Input: part model. Units: mm. Frame: model coordinates. A direction names the side the tool comes from. Round coordinates to 2 decimals unless told otherwise and drop trailing zeros. Loops run counter-clockwise (first coordinate to the right, second up) from the corner with the lowest first, then second, coordinate; pieces in that order, holes last.
(1) Cut plane C-C, the plane y = 0. Output: boundary loops of the cut face in (x, z).
(2) Line query: line 1 (Y direction, x = 0.6, z = 0); line 2 (Z direction, x = -1.5, y = 0.5); line 3 (Y direction, x = -1.5, z = -290). Output: solid intervals per line, ascending.
(3) First-contact query: pin 1 Ø2 at (x, z) = (0, -53) entering from +Y; pin 2 Ø6 at (x, z) = (0.5, -205.5) entering from +Y; pin 3 Ø3 at (x, y) = (-0.5, -20.5) entering from +Z. Flat tips, straight axial feed; report the tip coordinate or a pass-through.
(4) Access query for faces 3 (the face through (0.077, -99.847, -256.535)), 4 (the face through (3.007, -2.733, 116.812)), 5 (the face through (-2.97, 1.37, -566.71)), 6 (the face through (-0.04, -91.19, -255.66)). Directions: +Z, -Z, +X, -X, +Y, -Y. A direction counts if a zero-diameter tool reaches every point of the face in a straight line with its end or side. Return the directions, or none.
(5) Cut plane B-B, the plane z = 0. Output: boundary loops of the cut face in (x, y).
(6) Cut plane A-A, the plane x = 1. Output: boundary loops of the cut face in (y, z), and give its area (3 significant figures).
(7) Draft query along Z for faces 1 (the face through (0.08, 99.15, -263.47)), 2 (the face through (-2.97, -2.73, 116.69)). Return one class per face: released by +Z, released by -Z, zero draft, split by the parting line, or undercut.
from build123d import *


with BuildPart() as part:
    # 扫描1: sweep along a path in 草图1
    with BuildLine(Plane(origin=(0, 0, 0), x_dir=(0, 0, -1), z_dir=(1, 0, 0))) as sweep_1_path:
        Line((12.5, 124.373429638), (507.5, 74.624057783))
        ThreePointArc((507.5, 74.624057783), (575, 0), (507.5, -74.624057783))
        Line((507.5, -74.624057783), (12.5, -124.373429638))
        ThreePointArc((12.5, -124.373429638), (-125, 0), (12.5, 124.373429638))
    # 草图2 → 扫描1 (sweep)
    with BuildSketch(Plane.XY):
        Polygon((-5.5, 125), (5.5, 125), (2.840143071, 116.3), (-2.840143071, 116.3), align=None)
    sweep(path=sweep_1_path.line)


solid = part.part
Reported:
1. outline: (-5.5, -575) - (5.5, -575) - (2.84, -566.3) - (-2.84, -566.3) - close; (-5.5, 125) - (-2.84, 116.3) - (2.84, 116.3) - (5.5, 125) - close
2. line 1: y = -125 to -116.3, 116.3 to 125
2. line 2: z = -575 to -566.3, 116.3 to 125
2. line 3: y = -96.48 to -87.74, 87.74 to 96.48
3. pin 1: stops at y = 120.4
3. pin 2: stops at y = 105.28
3. pin 3: stops at z = 123.55
4. face 3: -Z, +X, -X, -Y
4. face 4: +X
4. face 5: -X
4. face 6: +X, -X
5. outline: (-5.5, -125) - (5.5, -125) - (2.84, -116.3) - (-2.84, -116.3) - close; (-5.5, 125) - (-2.84, 116.3) - (2.84, 116.3) - (5.5, 125) - close
6. outline: (-124.37, -12.5) - (-74.62, -507.5) arc R75 ccw to (74.62, -507.5) - (124.37, -12.5) arc R125 ccw (long way) to start; hole (-115.72, -11.63) - (-65.97, -506.63) arc R66.3 ccw to (65.97, -506.63) - (115.72, -11.63) arc R116.3 ccw (long way) to start
6. area: 14,000 mm2
7. face 1: released by -Z
7. face 2: undercut
